Could you check a few things on this model? Use its own coordinates, in mm. A direction names the side the tool comes from. Coordinates: 2 decimals unless noted, no trailing zeros. Write each loop counter-clockwise with the first axis right and the second up, starting at its lowest first coordinate (ties: lowest second). Pieces come first, ordered by that corner, then holes. Notation, with made-up numbers: (-29, 40.25) - (-1, 40.25) arc R32 cw to (-1, 71.25) - close; hole circle Ø6 at (66, -16.5). An arc over 180 degrees is marked (long way). Answer as a JSON object with one key per item and string values. Group by question number.
1) If we section it at D-D (z = -20): Write out the boundary of the cut face in (x, y).
2) Will these pins go through, and if not, where does the flat tip stop? pin 1 Ø1.8 at (y, z) = (9.5, -11.5) entering from +X; pin 2 Ø5 at (x, y) = (-43.5, 21.5) entering from +Z; pin 3 Ø1 at (x, z) = (-97.5, -29.5) entering from +Y.
3) If we section it at B-B (z = -45): Write out the boundary of the cut face in (x, y), plus the area to 3 significant figures.
4) If we section it at A-A (x = -40): Write out the boundary of the cut face in (y, z), plus the area to 3 significant figures.
5) If we section it at C-C (y = 20): Write out the boundary of the cut face in (x, z), plus the area to 3 significant figures.
6) Please list where these lines run through material, in increasing order: line 1 along Z through (x, y) = (-37, 11); line 2 along X through (y, z) = (24, -44); line 3 along Y through (x, z) = (-74, -24).
7) We'd pull the mould along Y, two halves only. Please class faces 1 (the cylindrical face through (-103.716, 16.222, -14.927)), 2 (the flat face through (-21.912, 1, -30)), 3 (the flat face through (-66, 30, -27)): released by +Y, released by -Y, zero draft, split by the parting line, or undercut.
8) On a 3-axis mill with a long thin cutter (end or side, diameter ignored), from which of +Z, -Z, +X, -X, +Y, -Y can I reach the whole of each face in a straight line? I mean faces 4 (the flat face through (-89.693, 16.057, -35.781)), 5 (the flat face through (-107, 2, -12)), 6 (the flat face through (-104.056, 15, -12)). Say none if no direction works.
```python
from build123d import *

# Parameters (mm, degrees)
BOSS_EXTRUDE3_DEPTH  = 30
SKETCH6_W            = 25
SKETCH6_H            = 23
CUT_EXTRUDE1_DEPTH   = 86
SKETCH7_W            = 25
SKETCH7_H            = 5
CUT_EXTRUDE2_DEPTH   = 7.5
SKETCH8_W            = 25
SKETCH8_H            = 2
CUT_EXTRUDE3_DEPTH   = 1
SKETCH9_R            = 19
CUT_EXTRUDE4_DEPTH   = 5
BOSS_EXTRUDE4_DEPTH  = 30
SKETCH10_W           = 1.856561782
SKETCH10_H           = 30
BOSS_EXTRUDE5_DEPTH  = 3
BOSS_EXTRUDE6_DEPTH  = 30
SKETCH11_W           = 2.5
SKETCH11_H           = 23
CUT_EXTRUDE5_DEPTH   = 34.579503854
SKETCH12_W           = 29.135235428
SKETCH12_H           = 25
CUT_EXTRUDE6_DEPTH   = 3.5
SKETCH13_W           = 19.135235428
SKETCH13_H           = 5
CUT_EXTRUDE7_DEPTH   = 3.5
SKETCH14_W           = 29.135235428
SKETCH14_H           = 4
BOSS_EXTRUDE7_DEPTH  = 2
SKETCH16_W           = 29.135235428
SKETCH16_H           = 1.5
BOSS_EXTRUDE8_DEPTH  = 2
SKETCH17_W           = 2.551467674
SKETCH17_H           = 30
BOSS_EXTRUDE9_DEPTH  = 5
BOSS_EXTRUDE10_REACH = 85.266
SKETCH18_W           = 29.135235428
SKETCH18_H           = 2.5
SKETCH19_W           = 2.48850009
SKETCH19_H           = 23
BOSS_EXTRUDE11_DEPTH = 2
CUT_EXTRUDE8_START   = -2.4885
SKETCH20_W           = 2
SKETCH20_H           = 23
CUT_EXTRUDE8_DEPTH   = 21.736568
BOSS_EXTRUDE12_REACH = 82.714
SKETCH21_W           = 2.023287715
SKETCH21_H           = 27.5


with BuildPart() as part:
    # Sketch2 → Boss-Extrude3 (new body)
    with BuildSketch(Plane(origin=(0, 0, 0), x_dir=(1, 0, 0), z_dir=(0, 1, 0))):
        Polygon((-105.912162162, 13.018018018), (-20.912162162, 13.018018018), (-20.912162162, 48.018018018), (-75.912162162, 48.018018018), align=None)
    extrude(amount=BOSS_EXTRUDE3_DEPTH)

    # Sketch6 → Cut-Extrude1 (cut, through all)
    with BuildSketch(Plane(origin=(-20.912162162, 0, 0), x_dir=(0, 0, -1), z_dir=(1, 0, 0))):
        with Locations((30.518018018, 13.5)):
            Rectangle(SKETCH6_W, SKETCH6_H)
    extrude(amount=-CUT_EXTRUDE1_DEPTH, mode=Mode.SUBTRACT)

    # Sketch7 → Cut-Extrude2 (cut)
    with BuildSketch(Plane(origin=(-20.912162162, 0, 0), x_dir=(0, 0, -1), z_dir=(1, 0, 0))):
        with Locations((30.518018018, 27.5)):
            Rectangle(SKETCH7_W, SKETCH7_H)
    extrude(amount=-CUT_EXTRUDE2_DEPTH, mode=Mode.SUBTRACT)

    # Sketch8 → Cut-Extrude3 (cut)
    with BuildSketch(Plane(origin=(-20.912162162, 0, 0), x_dir=(0, 0, -1), z_dir=(1, 0, 0))):
        with Locations((30.518018018, 1)):
            Rectangle(SKETCH8_W, SKETCH8_H)
    extrude(amount=-CUT_EXTRUDE3_DEPTH, mode=Mode.SUBTRACT)

    # Sketch9 → Cut-Extrude4 (cut)
    with BuildSketch(Plane.XY.offset(-13.018018018)):
        with Locations((-84.912162162, 13.5)):
            Circle(SKETCH9_R)
    extrude(amount=-CUT_EXTRUDE4_DEPTH, mode=Mode.SUBTRACT)

    # Sketch3 → Boss-Extrude4 (add)
    with BuildSketch(Plane(origin=(0, 0, 0), x_dir=(1, 0, 0), z_dir=(0, 1, 0))):
        Polygon((-106.412808957, 7.383361614), (-110.17791555, 11.88278259), (-79.204856611, 48.018018018), (-75.912162162, 48.018018018), (-105.912162162, 13.018018018), (-103.345157358, 9.950366419), align=None)
    extrude(amount=BOSS_EXTRUDE4_DEPTH)

    # Sketch10 → Boss-Extrude5 (add)
    with BuildSketch(Plane.XY.offset(-13.018018018)):
        with Locations((-104.983881271, 15)):
            Rectangle(SKETCH10_W, SKETCH10_H)
    extrude(amount=BOSS_EXTRUDE5_DEPTH)

    # Sketch4 → Boss-Extrude6 (add)
    with BuildSketch(Plane(origin=(0, 0, 0), x_dir=(1, 0, 0), z_dir=(0, 1, 0))):
        Polygon((-110.17791555, 11.88278259), (-110.17791555, 48.018018018), (-104.17791555, 48.018018018), (-104.17791555, 18.88278259), align=None)
    extrude(amount=BOSS_EXTRUDE6_DEPTH)

    # Sketch11 → Cut-Extrude5 (cut, through all)
    with BuildSketch(Plane(origin=(-47.459390138, 0, -56.715466139), x_dir=(0.7669129, 0, -0.641751201), z_dir=(0.641751201, 0, 0.7669129))):
        with Locations((-74.121074711, 13.5)):
            Rectangle(SKETCH11_W, SKETCH11_H)
    extrude(amount=-CUT_EXTRUDE5_DEPTH, mode=Mode.SUBTRACT)

    # Sketch12 → Cut-Extrude6 (cut)
    with BuildSketch(Plane(origin=(-104.17791555, 0, 0), x_dir=(0, 0, -1), z_dir=(1, 0, 0))):
        with Locations((33.450400304, 15)):
            Rectangle(SKETCH12_W, SKETCH12_H)
    extrude(amount=-CUT_EXTRUDE6_DEPTH, mode=Mode.SUBTRACT)

    # Sketch13 → Cut-Extrude7 (cut, through all)
    with BuildSketch(Plane(origin=(-107.67791555, 0, 0), x_dir=(0, 0, -1), z_dir=(1, 0, 0))):
        with Locations((38.450400304, 15)):
            Rectangle(SKETCH13_W, SKETCH13_H)
    extrude(amount=-CUT_EXTRUDE7_DEPTH, mode=Mode.SUBTRACT)

    # Sketch14 → Boss-Extrude7 (add)
    with BuildSketch(Plane(origin=(-107.67791555, 0, 0), x_dir=(0, 0, -1), z_dir=(1, 0, 0))):
        with Locations((33.450400304, 25.5)):
            Rectangle(SKETCH14_W, SKETCH14_H)
    extrude(amount=BOSS_EXTRUDE7_DEPTH)

    # Sketch16 → Boss-Extrude8 (add)
    with BuildSketch(Plane(origin=(-107.67791555, 0, 0), x_dir=(0, 0, -1), z_dir=(1, 0, 0))):
        with Locations((33.450400304, 3.25)):
            Rectangle(SKETCH16_W, SKETCH16_H)
    extrude(amount=BOSS_EXTRUDE8_DEPTH)

    # Sketch17 → Boss-Extrude9 (add)
    with BuildSketch(Plane(origin=(0, 0, -18.88278259), x_dir=(-1, 0, 0), z_dir=(0, 0, -1))):
        with Locations((102.902181713, 15)):
            Rectangle(SKETCH17_W, SKETCH17_H)
    extrude(amount=BOSS_EXTRUDE9_DEPTH)

    # Boss-Extrude10: up to this face of the body (flat: up to its plane)
    boss_extrude10_end = Plane(part.part.faces().sort_by_distance((-90.415652244, 15, -34.938756447))[0])
    # Sketch18 → Boss-Extrude10 (add, up to the picked face)
    with BuildSketch(Plane(origin=(-104.17791555, 0, 0), x_dir=(0, 0, -1), z_dir=(1, 0, 0)), mode=Mode.PRIVATE) as boss_extrude10_sk1:
        with Locations((33.450400304, 1.25)):
            Rectangle(SKETCH18_W, SKETCH18_H)
    boss_extrude10_tool1 = split(extrude(boss_extrude10_sk1.sketch, amount=BOSS_EXTRUDE10_REACH, mode=Mode.PRIVATE), bisect_by=boss_extrude10_end, keep=Keep.BOTH, mode=Mode.PRIVATE)
    add(boss_extrude10_tool1.solids().sort_by_distance((-104.177916, 1.25, -33.4504))[0])

    # Sketch19 → Boss-Extrude11 (add)
    with BuildSketch(Plane(origin=(-67.487678855, 0, -57.846581876), x_dir=(0.650791373, 0, -0.759256602), z_dir=(0.759256602, 0, 0.650791373))):
        with Locations((-31.723015124, 13.5)):
            Rectangle(SKETCH19_W, SKETCH19_H)
    extrude(amount=BOSS_EXTRUDE11_DEPTH)

    # Sketch20 → Cut-Extrude8 (cut)
    with BuildSketch(Plane(origin=(-19.835317387, 0, 23.141203618), x_dir=(-0.759256602, 0, -0.650791373), z_dir=(0.650791373, 0, -0.759256602)).offset(CUT_EXTRUDE8_START)):
        with Locations((87.886522218, 13.5)):
            Rectangle(SKETCH20_W, SKETCH20_H)
    extrude(amount=CUT_EXTRUDE8_DEPTH, mode=Mode.SUBTRACT)

    # Boss-Extrude12: up to this face of the body (flat: up to its plane)
    boss_extrude12_end = Plane(part.part.faces().sort_by_distance((-90.415652244, 16.25, -34.938756447))[0])
    # Sketch21 → Boss-Extrude12 (add, up to the picked face)
    with BuildSketch(Plane(origin=(-101.626447876, 0, 0), x_dir=(0, 0, -1), z_dir=(1, 0, 0)), mode=Mode.PRIVATE) as boss_extrude12_sk1:
        with Locations((22.871138733, 16.25)):
            Rectangle(SKETCH21_W, SKETCH21_H)
    boss_extrude12_tool1 = split(extrude(boss_extrude12_sk1.sketch, amount=BOSS_EXTRUDE12_REACH, mode=Mode.PRIVATE), bisect_by=boss_extrude12_end, keep=Keep.BOTH, mode=Mode.PRIVATE)
    add(boss_extrude12_tool1.solids().sort_by_distance((-101.626448, 16.25, -22.871139))[0])


solid = part.part
```
Here are the results:
{
 "1": {"outline": "(-110.18, 0) - (-21.91, 0) - (-21.91, 2) - (-99.93, 2) - (-99.93, 25) - (-28.41, 25) - (-28.41, 30) - (-110.18, 30) - close; hole (-107.68, 4) - (-105.68, 4) - (-105.68, 2.5) - (-104.18, 2.5) - (-104.18, 27.5) - (-105.68, 27.5) - (-105.68, 23.5) - (-107.68, 23.5) - close"},
 "2": {"pin 1": "stops at x = -104.06", "pin 2": "stops at z = -13.02", "pin 3": "stops at y = 2.5"},
 "3": {"outline": "(-110.18, 0) - (-20.91, 0) - (-20.91, 30) - (-81.79, 30) - (-81.79, 2.5) - (-105.68, 2.5) - (-105.68, 4) - (-107.68, 4) - (-107.68, 12.5) - (-110.18, 12.5) - close; (-110.18, 17.5) - (-107.68, 17.5) - (-107.68, 23.5) - (-105.68, 23.5) - (-105.68, 27.5) - (-104.18, 27.5) - (-104.18, 30) - (-110.18, 30) - close; hole (-78.5, 2) - (-75.86, 2) - (-75.86, 25) - (-78.5, 25) - close", "area": "1,910 mm²"},
 "4": {"outline": "(0, -48.02) - (30, -48.02) - (30, -13.02) - (0, -13.02) - close; hole (2, -43.02) - (25, -43.02) - (25, -18.02) - (2, -18.02) - close", "area": "475 mm²"},
 "5": {"outline": "(-110.18, -48.02) - (-107.68, -48.02) - (-107.68, -18.88) - (-104.18, -18.88) - (-104.18, -23.88) - (-99.89, -23.88) - (-79.2, -48.02) - (-75.91, -48.02) - (-102.77, -16.69) - (-102.77, -13.02) - (-104.06, -13.02) - (-104.06, -10.8) - (-110.18, -18.12) - close; (-110.18, -14.22) - (-105.26, -8.35) - (-106.41, -7.38) - (-110.18, -11.88) - close; (-77.56, -43.02) - (-73.28, -48.02) - (-20.91, -48.02) - (-20.91, -43.02) - close; (-67.06, -18.02) - (-20.91, -18.02) - (-20.91, -13.02) - (-67.06, -13.02) - close", "area": "730 mm²"},
 "6": {"line 1": "z = -48.02 to -43.02, -18.02 to -13.02", "line 2": "x = -110.18 to -105.68, -82.65 to -79.36, -76.72 to -20.91", "line 3": "y = 0 to 2, 25 to 30"},
 "7": {"face 1": "undercut", "face 2": "zero draft", "face 3": "released by +Y"},
 "8": {"face 4": "-Z, +Y", "face 5": "none", "face 6": "+X, +Y, -Y"}
}
